from build123d import *

# Parameters (mm, degrees)
PAD002_DEPTH    = 5
PAD001_DEPTH    = 20
PAD003_DEPTH    = 5
PAD_DEPTH       = 14.5
SKETCH009_R     = 10
POCKET_DEPTH    = 134.001
SKETCH010_R     = 10
POCKET001_DEPTH = 17.001
SKETCH011_R     = 10
POCKET002_DEPTH = 17.001
FILLET_R        = 2


with BuildPart() as revolution001:
    # Sketch005 → Revolution001 (revolve)
    with BuildSketch(Plane.YZ):
        Polygon((20, 70), (20, 87.5), (22.5, 90), (37.5, 90), (40, 87.5), (40, 70), align=None)
    revolve(axis=Axis((0, 20, 70), (0, -1, 0)))


with BuildPart() as pad002:
    # Sketch002 → Pad002 (new body, symmetric)
    with BuildSketch(Plane.YZ):
        Polygon((-37.5, 49.5), (-37.5, 14.5), (-49.5, 14.5), align=None)
        Polygon((37.5, 14.5), (49.5, 14.5), (37.5, 49.5), align=None)
    extrude(amount=PAD002_DEPTH, both=True)


with BuildPart() as pad001:
    # Sketch001 → Pad001 (new body, symmetric)
    with BuildSketch(Plane.YZ):
        Polygon((-37.5, 0), (-37.5, 70), (-22.5, 70), (-22.5, 27), (22.5, 27), (22.5, 70), (37.5, 70), (37.5, 0), align=None)
    extrude(amount=PAD001_DEPTH, both=True)


with BuildPart() as revolution004:
    # Sketch008 → Revolution004 (revolve)
    with BuildSketch(Plane.XZ):
        Polygon((55, 14.5), (75, 14.5), (75, 17), (57.5, 17), align=None)
    revolve(axis=Axis((75, 0, 14.5), (0, 0, -1)))


with BuildPart() as pad003:
    # Sketch003 → Pad003 (new body, symmetric)
    with BuildSketch(Plane.XZ):
        Polygon((20, 27), (20, 14.5), (54, 14.5), (26, 27), align=None)
    extrude(amount=PAD003_DEPTH, both=True)


with BuildPart() as revolution003:
    # Sketch007 → Revolution003 (revolve)
    with BuildSketch(Plane.YZ):
        Polygon((50, 14.5), (70, 14.5), (70, 17), (52.5, 17), align=None)
    revolve(axis=Axis((0, 70, 14.5), (0, 0, -1)))


with BuildPart() as revolution002:
    # Sketch006 → Revolution002 (revolve)
    with BuildSketch(Plane.YZ):
        Polygon((-90, 14.5), (-70, 14.5), (-70, 17), (-87.5, 17), align=None)
    revolve(axis=Axis((0, -70, 14.132615), (0, 0, -1)))


with BuildPart() as revolution:
    # Sketch004 → Revolution (revolve)
    with BuildSketch(Plane.YZ):
        Polygon((-40, 70), (-40, 87.5), (-37.5, 90), (-22.5, 90), (-20, 87.5), (-20, 70), align=None)
    revolve(axis=Axis((0, -20, 70), (0, 1, 0)))


with BuildPart() as fillet_body:
    # Sketch → Pad (new body)
    with BuildSketch(Plane.XY):
        with BuildLine():
            Line((-24, 70), (-24, -70.000001))
            ThreePointArc((-24, -70.000001), (1e-06, -94), (24, -70))
            Line((24, -70), (24, -25))
            Line((24, -25), (75, -25))
            ThreePointArc((75, -25), (100, 0), (74.999999, 25))
            Line((24, 25), (74.999999, 25))
            Line((24, 70), (24, 25))
            ThreePointArc((24, 70), (0, 94), (-24, 70))
        make_face()
    extrude(amount=PAD_DEPTH)

    # Fusion: union Revolution001, Pad002, Pad001, Revolution004, Pad003, Revolution003, Revolution002, Revolution
    add(revolution001.part)
    add(pad002.part)
    add(pad001.part)
    add(revolution004.part)
    add(pad003.part)
    add(revolution003.part)
    add(revolution002.part)
    add(revolution.part)

    # Sketch009 → Pocket (cut, through all)
    with BuildSketch(Plane.XZ.offset(40)):
        with Locations((0, 70)):
            Circle(SKETCH009_R)
    extrude(amount=-POCKET_DEPTH, mode=Mode.SUBTRACT)

    # Sketch010 → Pocket001 (cut, through all)
    with BuildSketch(Plane.XY.offset(17)):
        with Locations((0, 70)):
            Circle(SKETCH010_R)
        with Locations((0, -70)):
            Circle(SKETCH010_R)
    extrude(amount=-POCKET001_DEPTH, mode=Mode.SUBTRACT)

    # Sketch011 → Pocket002 (cut, through all)
    with BuildSketch(Plane.XY.offset(17)):
        with Locations((75, 0)):
            Circle(SKETCH011_R)
    extrude(amount=-POCKET002_DEPTH, mode=Mode.SUBTRACT)

    # Fillet
    fillet_edges = [fillet_body.edges().sort_by_distance(p)[0] for p in [
        (0, 22.5, 27),
        (24, -25, 7.25),
        (24, 25, 7.25),
        (0, -22.5, 27),
    ]]
    fillet(fillet_edges, radius=FILLET_R)


solid = fillet_body.part
Design review of the part built by this model. Coordinates are the model's own, in mm. A direction names the side the tool comes from. Give positions to 0.01 mm unless a question says otherwise; leave off trailing zeros. Loops run counter-clockwise (first coordinate to the right, second up) from the corner with the lowest first, then second, coordinate; pieces in that order, holes last. Notation, with made-up numbers: (64.5, -39) -> (106.5, -39) arc R17 cw to (106.5, -7) -> close; hole circle Ø1 at (-36.5, 38). An arc over 180 degrees is marked (long way). One line per question, with ' | ' between items. Start each with the question number.
(1) We need section C-C (x = 2.5). State how many separate pieces and enclosed holes the cut face has, and give its area (3 significant figures).
(2) Insertion check: P1, Ø6, axis at y = 45.5, z = 31.5, coming from the -X side; P2, Ø10, axis at x = 41, y = -2, coming from the +Z side; P3, Ø12, axis at x = -6.5, z = 44.5, coming from the +Y side; P4, Ø12, axis at x = 0, y = -70, coming from the +Z side. Each pin has a flat end and moves straight along its axis. Give the tip position at first contact, or say it passes through.
(3) For faces 1 (the face through (-8, -20, 78)), 2 (the face through (8, -62, 17)), 3 (the face through (-5, 41, 24)), list the 3-axis set-ups (+Z, -Z, +X, -X, +Y, -Y) from which the entire face can be reached by the end or side of a thin tool; tool diameter is ignored.
(4) For line 1 (Y direction, x = 0, z = 5); line 2 (Z direction, x = 0, y = 28.75); line 3 (Y direction, x = -10, z = 64), list the stretches that pass through material, from the lowest coordinate up.
(5) Draft analysis for pull direction X (two halves, no side actions). For faces 4 (the face through (5.38, 29.86, 78.43)), 5 (the face through (24, -7, 14.5)), 6 (the face through (99.994, -0.55, 7.148)), 7 (the face through (8, 20, 62)), state which applies: +X half, -X half, draft (parallel to the pull), parting line (faces both ways), or undercut.
(6) We need section A-A (y = 0). State the section outline as (x, z) points.
(7) We need section B-B (x = 47.5). State the section outline as (y, z) points.
The answers:
1) separate pieces: 5 | enclosed holes: 0 | area: 5,090 mm^2
2) P1: stops at x = -5 | P2: stops at z = 22.54 | P3: stops at y = 41.21 | P4: passes through
3) face 1: +Z, +X, -X | face 2: +Z, +X, -X, -Y | face 3: -X
4) line 1: y = -94 to -80, -60 to 60, 80 to 94 | line 2: z = 0 to 60, 80 to 90 | line 3: y = -40 to -20, 20 to 40
5) face 4: undercut | face 5: undercut | face 6: +X half | face 7: draft
6) outline: (-24, 0) -> (65, 0) -> (65, 17) -> (57.5, 17) -> (55, 14.5) -> (54, 14.5) -> (26, 27) -> (-20, 27) -> (-20, 14.5) -> (-24, 14.5) -> close; (85, 0) -> (100, 0) -> (100, 14.5) -> (95, 14.5) -> (92.5, 17) -> (85, 17) -> close
7) outline: (-25, 0) -> (25, 0) -> (25, 14.5) -> (5, 14.5) -> (5, 17.4) -> (-5, 17.4) -> (-5, 14.5) -> (-25, 14.5) -> close
